```python
from build123d import *

# Parameters (mm, degrees)
SKETCH_1_W          = 12
SKETCH_1_H          = 2
EXTRUDE_1_DEPTH     = 4
EXTRUDE_2_DEPTH     = 4
EXTRUDE_4_DEPTH     = 4
SKETCH_8_R          = 0.5
CUT_EXTRUDE_1_DEPTH = 10
SKETCH_9_R          = 0.4
CUT_EXTRUDE_2_DEPTH = 10
SCALE_1_SCALE       = 2.454545455
FILLET_1_R          = 1
CHAMFER_1_SIZE      = 0.3
FILLET_2_R          = 1
FILLET_3_R          = 10


with BuildPart() as part:
    # 草图1 → 凸台-拉伸1 (new body)
    with BuildSketch(Plane(origin=(0, 0, 0), x_dir=(0, 0, -1), z_dir=(1, 0, 0))):
        with Locations((-7.174242424, 4.674378087)):
            Rectangle(SKETCH_1_W, SKETCH_1_H)
    extrude(amount=EXTRUDE_1_DEPTH)

    # 草图4 → 凸台-拉伸2 (add)
    with BuildSketch(Plane(origin=(4, 0, 0), x_dir=(0, 0, -1), z_dir=(1, 0, 0))):
        Polygon((-1.174242424, 5.674378087), (-1.174242424, 3.674378087), (7.484707821, -4.633604859), (7.484707821, -2.633604859), align=None)
    extrude(amount=-EXTRUDE_2_DEPTH)

    # 草图7 → 凸台-拉伸4 (add)
    with BuildSketch(Plane(origin=(4, 0, 0), x_dir=(0, 0, -1), z_dir=(1, 0, 0))):
        with BuildLine():
            Line((-13.174242424, 5.674378087), (-13.174242424, 3.674378087))
            ThreePointArc((-13.174242424, 3.674378087), (-14.174242424, 4.674378087), (-13.174242424, 5.674378087))
        make_face()
    extrude(amount=-EXTRUDE_4_DEPTH)

    # 草图8 → 切除-拉伸1 (cut)
    with BuildSketch(Plane(origin=(4, 0, 0), x_dir=(0, 0, -1), z_dir=(1, 0, 0))):
        with Locations((-12.981538842, 4.72790686)):
            Circle(SKETCH_8_R)
    extrude(amount=-CUT_EXTRUDE_1_DEPTH, mode=Mode.SUBTRACT)

    # 草图9 → 切除-拉伸2 (cut)
    with BuildSketch(Plane(origin=(4, 0, 0), x_dir=(0, 0, -1), z_dir=(1, 0, 0))):
        with Locations((6.619490877, -2.882976322)):
            Circle(SKETCH_9_R)
    extrude(amount=-CUT_EXTRUDE_2_DEPTH, mode=Mode.SUBTRACT)


with BuildPart() as part_1:
    # 缩放比例1: scaled about (2, 3.035419998, 3.173801188)
    add(part.part.scale(SCALE_1_SCALE).moved(Location((-2.909090909, -4.415156361, -4.616438092))))

    # 圆角1
    fillet_1_edges = [part_1.edges().sort_by_distance(p)[0] for p in [
        (2, -10.879459197, -22.987993653),
        (2, -15.788550106, -22.987993653),
    ]]
    fillet(fillet_1_edges, radius=FILLET_1_R)

    # 倒角1
    chamfer_1_edges = [part_1.edges().sort_by_distance(p)[0] for p in [
        (-2.909090909, -4.780520326, -11.514934214),
        (6.909090909, 4.603771672, 12.993066041),
        (6.909090909, -4.780520326, -11.514934214),
        (-2.909090909, 7.058317127, 30.174884222),
        (6.909090909, 7.058317127, 30.174884222),
        (6.909090909, 7.189705933, 28.474611794),
        (6.909090909, -11.491552788, -19.882461153),
        (6.909090909, -12.374536967, -22.987993653),
        (-2.909090909, -12.374536967, -22.987993653),
        (-2.909090909, 4.603771672, 12.993066041),
        (6.909090909, -0.535699514, -12.207266126),
        (6.909090909, -14.36310593, -22.380210486),
        (6.909090909, -10.913623963, -22.907866447),
        (-2.909090909, -0.535699514, -12.207266126),
        (-2.909090909, -14.36310593, -22.380210486),
        (-2.909090909, -10.913623963, -22.907866447),
        (-2.909090909, 9.512862581, 12.993066041),
        (6.909090909, 9.512862581, 12.993066041),
    ]]
    chamfer(chamfer_1_edges, length=CHAMFER_1_SIZE)

    # 圆角2
    fillet_2_edges = [part_1.edges().sort_by_distance(p)[0] for p in [
        (2, 9.512862581, -1.734206687),
    ]]
    fillet(fillet_2_edges, radius=FILLET_2_R)

    # 圆角3
    fillet_3_edges = [part_1.edges().sort_by_distance(p)[0] for p in [
        (2, 4.603771672, -1.734206687),
    ]]
    fillet(fillet_3_edges, radius=FILLET_3_R)


solid = part_1.part
```
Geometry: final body of the model. Coordinates: model frame, mm. A direction names the side the tool comes from. Give positions to 0.01 mm unless a question says otherwise; leave off trailing zeros. Loops run counter-clockwise (first coordinate to the right, second up) from the corner with the lowest first, then second, coordinate; pieces in that order, holes last. Notation, with made-up numbers: (29.5, -20.75) -> (85.5, -20.75) arc R18 cw to (85.5, 2.25) -> close; hole circle Ø6 at (-37, 44). An arc over 180 degrees is marked (long way). Return JSON: item names as keys, results as strings.
Item 1: Pin query (flat end, axial travel): P1, Ø3, axis at x = 0, z = 17, coming from the -Y side; P2, Ø3, axis at y = 7.19, z = 27.25, coming from the +X side; P3, Ø1.2, axis at y = -11.49, z = -20.86, coming from the +X side; P4, Ø5, axis at x = 0, z = -9.5, coming from the -Y side. Return the tip coordinate at first contact, or that it passes through.
Filled in:
{"P1": "y = 4.6", "P2": "x = 6.88", "P3": "through", "P4": "y = -5.25"}
Item 2: Access query for faces 1 (the flat face through (2, -12, -22.988)), 2 (the flat face through (6.736, 4.731, 11.906)), 3 (the flat face through (-2.746, 4.741, 12.726)). Directions: +Z, -Z, +X, -X, +Y, -Y. A direction counts if a zero-diameter tool reaches every point of the face in a straight line with its end or side. Return the directions, or none.
Filled in:
{"face 1": "-Z, +X, -X, +Y, -Y", "face 2": "+Z, +X, -Y", "face 3": "+Z, -X, -Y"}
Item 3: Section A-A, the plane z = 13. Output: boundary loops of the cut face in (x, y).
Filled in:
{"outline": "(-2.91, 4.9) -> (-2.61, 4.6) -> (6.61, 4.6) -> (6.91, 4.9) -> (6.91, 9.21) -> (6.61, 9.51) -> (-2.61, 9.51) -> (-2.91, 9.21) -> close"}
Item 4: Section B-B, the plane x = -0.5. Output: boundary loops of the cut face in (y, z).
Filled in:
{"outline": "(-14.16, -21.3) arc R1 ccw to (-13.44, -22.99) -> (-11.31, -22.99) arc R1 ccw to (-10.58, -22.68) -> (9.23, -2.02) arc R1 ccw to (9.51, -1.33) -> (9.51, 27.72) arc R2.45 ccw to (4.6, 27.72) -> (4.6, 2.29) arc R10 cw to (1.82, -4.64) -> close; hole circle Ø1.96 at (-11.49, -20.86); hole circle Ø2.45 at (7.19, 27.25)"}
Item 5: Line query: line 1 (Y direction, x = 1.5, z = 11.5); line 2 (Z direction, x = 6, y = 7.5); line 3 (Z direction, x = 1.75, y = 6.5). Output: solid intervals per line, ascending.
Filled in:
{"line 1": "4.6 to 9.51", "line 2": "-3.83 to 26.06, 28.43 to 30.13", "line 3": "-4.87 to 26.23, 28.26 to 30.11"}
Item 6: Section C-C, the plane y = 3. Output: boundary loops of the cut face in (x, z).
Filled in:
{"outline": "(-2.91, -8.09) -> (-2.61, -8.52) -> (6.61, -8.52) -> (6.91, -8.09) -> (6.91, -3.84) -> (6.43, -3.14) -> (-2.43, -3.14) -> (-2.91, -3.84) -> close"}
Item 7: Mould query, pull axis Y, two halves, no side actions, for faces 4 (the flat face through (-2.746, -4.508, -11.429)), 5 (the conical face through (-2.795, 7.008, 29.989)), 6 (the cylindrical face through (1.92, 5.99, 27.51)). Classes: released by +Y, released by -Y, zero draft, split by the parting line, or undercut.
Filled in:
{"face 4": "released by -Y", "face 5": "split by the parting line", "face 6": "undercut"}
